Work out the finished part from the listing and answer in its coordinate system (mm). Round coordinates to 2 decimals unless told otherwise and drop trailing zeros. Write each loop counter-clockwise with the first axis right and the second up, starting at its lowest first coordinate (ties: lowest second). Pieces come first, ordered by that corner, then holes.
1. A flat-ended cylindrical pin translates along its axis: pin 1 Ø12.5 at (x, z) = (-19.89, -11.5) entering from +Y. Find the tip coordinate at first contact, or state that the pin passes through.
2. Straight lines are drawn through the part: probe 1 along X at (y, z) = (5, -11.5); probe 2 along X at (y, z) = (5.75, -15); probe 3 along X at (y, z) = (4, -5.75). For each, find the intervals that lie inside material, in ascending order.
3. Find section D-D (x = -3.5). Write down the section's boundary in (y, z), and give its area (3 significant figures).
4. Find section C-C (y = 1). Write down the section's boundary in (x, z), and give its area (3 significant figures).
5. Determine the mould class of faces 1 (the face through (0.35, 4.82, -16.99)), 2 (the face through (0, 5, -22.997)), 3 (the face through (-6, 0, -12)) for opening direction Z: pulls with the +Z half, pulls with the -Z half, needs draft (parallel to the pull), parting line crosses it, or undercut.
6. Find section B-B (x = 4). Write down the section's boundary in (y, z), and give its area (3 significant figures).
7. Find section A-A (z = -11.5). Write down the section's boundary in (x, y), and give its area (3 significant figures).
```python
from build123d import *

# Parameters (mm, degrees)
EXTRUDE_1_DEPTH     = 9.5
FILLET_1_R          = 3
SKETCH_2_R          = 7.75
SKETCH_2_R_2        = 5.5
CUT_EXTRUDE_2_DEPTH = 10


with BuildPart() as part:
    # 草图1 → 凸台-拉伸1 (new body)
    with BuildSketch(Plane(origin=(0, 0, 0), x_dir=(1, 0, 0), z_dir=(0, 1, 0))):
        Polygon((0, 0), (-30, 0), (-30, 23), (-14, 23), (-14, 22.997077799), (14, 22.997077799), (14, 23), (30, 23), (30, 0), align=None)
    extrude(amount=EXTRUDE_1_DEPTH)

    # 圆角1
    # the kernel refuses this fillet: 3 mm, written as the material it adds along each edge
    with BuildSketch(Plane(origin=(14, 0, -22.997077799), x_dir=(-2.4315329398816435e-12, 0, -1.0), z_dir=(0, 1, 0))) as fillet_1_piece_1:
        with BuildLine():
            CenterArc((3, 0.132380758), FILLET_1_R, 180, 2.529107474)
            Line((0, 0.132380758), (0, 0))
            Line((0, 0), (0.002922201, 0))
        make_face()
    extrude(amount=9.5)
    with BuildSketch(Plane(origin=(-14, 0, -22.997077799), x_dir=(1, 0, 0), z_dir=(0, 1, 0))) as fillet_1_piece_2:
        with BuildLine():
            CenterArc((0.132380758, 3), FILLET_1_R, 267.470892526, 2.529107474)
            Line((0, 0.002922201), (0, 0))
            Line((0, 0), (0.132380758, 0))
        make_face()
    extrude(amount=9.5)
    # the kernel refuses this fillet: 3 mm, written as the material it takes off along each edge
    with BuildSketch(Plane(origin=(30, -7.5, -23), x_dir=(0, 0, 1), z_dir=(0, 1, 0))) as fillet_1_2_piece_1:
        with BuildLine():
            CenterArc((FILLET_1_R, -FILLET_1_R), FILLET_1_R, 90, 90)
            Line((0, -FILLET_1_R), (0, 0))
            Line((0, 0), (FILLET_1_R, 0))
        make_face()
    extrude(amount=24.5, mode=Mode.SUBTRACT)
    with BuildSketch(Plane(origin=(-30, -7.5, -23), x_dir=(0, 0, 1), z_dir=(0, 1, 0))) as fillet_1_2_piece_2:
        with BuildLine():
            CenterArc((FILLET_1_R, FILLET_1_R), FILLET_1_R, 180, 90)
            Line((0, FILLET_1_R), (0, 0))
            Line((0, 0), (FILLET_1_R, 0))
        make_face()
    extrude(amount=24.5, mode=Mode.SUBTRACT)

    # 草图2 → 切除-拉伸2 (cut)
    with BuildSketch(Plane(origin=(0, 9.5, 0), x_dir=(1, 0, 0), z_dir=(0, 1, 0))):
        with Locations(Location((20.11016513, 11.5, 0), (0, 0, 270))):
            Circle(SKETCH_2_R)
        with Locations(Location((-19.88983487, 11.5, 0), (0, 0, 270))):
            Circle(SKETCH_2_R)
        with Locations(Location((0.11016513, 11.497077799, 0), (0, 0, 270))):
            Circle(SKETCH_2_R_2)
    extrude(amount=-CUT_EXTRUDE_2_DEPTH, mode=Mode.SUBTRACT)


solid = part.part
```
Worked answers:
1. pin 1: passes through
2. probe 1: x = -30 to -27.64, -12.14 to -5.39, 5.61 to 12.36, 27.86 to 30
2. probe 2: x = -30 to -26.8, -12.98 to -4.13, 4.35 to 13.2, 27.02 to 30
2. probe 3: x = -30 to -25.09, -14.69 to 14.91, 25.31 to 30
3. outline: (0, -23) - (9.5, -23) - (9.5, -15.65) - (0, -15.65) - close; (0, -7.35) - (9.5, -7.35) - (9.5, 0) - (0, 0) - close
3. area: 140 mm2
4. outline: (-30, -20) arc R3 ccw to (-27, -23) - (-14, -23) arc R3 cw to (-13.87, -23) - (13.87, -23) arc R3 cw to (14, -23) - (27, -23) arc R3 ccw to (30, -20) - (30, 0) - (-30, 0) - close; hole circle Ø15.5 at (-19.89, -11.5); hole circle Ø11 at (0.11, -11.5); hole circle Ø15.5 at (20.11, -11.5)
4. area: 904 mm2
5. face 1: undercut
5. face 2: pulls with the -Z half
5. face 3: needs draft
6. outline: (0, -23) - (9.5, -23) - (9.5, -15.39) - (0, -15.39) - close; (0, -7.61) - (9.5, -7.61) - (9.5, 0) - (0, 0) - close
6. area: 145 mm2
7. outline: (-30, 0) - (-27.64, 0) - (-27.64, 9.5) - (-30, 9.5) - close; (-12.14, 0) - (-5.39, 0) - (-5.39, 9.5) - (-12.14, 9.5) - close; (5.61, 0) - (12.36, 0) - (12.36, 9.5) - (5.61, 9.5) - close; (27.86, 0) - (30, 0) - (30, 9.5) - (27.86, 9.5) - close
7. area: 171 mm2
